Here's the drawing with two shaded views (mm, measured from the low corner). I have some questions. Give positions to 0.01 mm unless a question says otherwise; leave off trailing zeros. Write each loop counter-clockwise with the first axis right and the second up, starting at its lowest first coordinate (ties: lowest second). Pieces come first, ordered by that corner, then holes. Notation, with made-up numbers: (1, 21.5) - (28, 21.5) arc R24 cw to (28, 43.5) - close; hole circle Ø2 at (22, 58.5). An arc over 180 degrees is marked (long way). Write item = value, one per line.
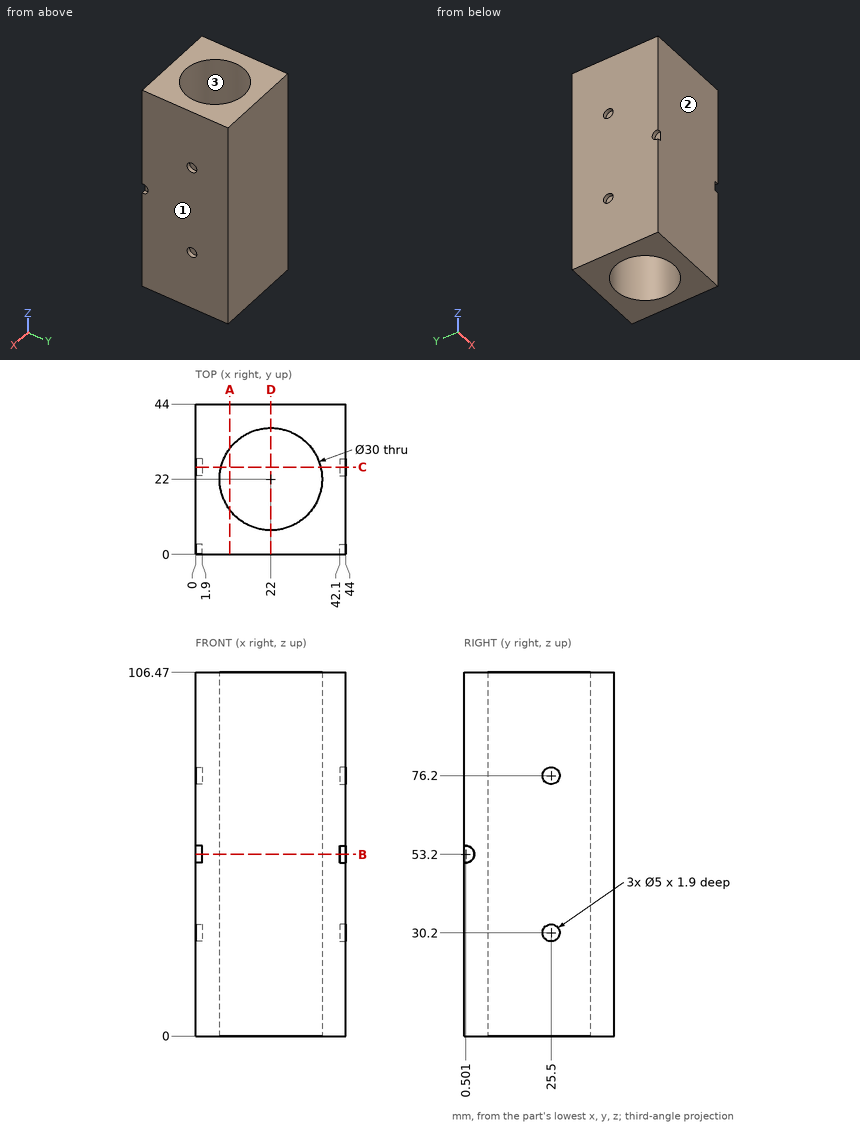
1. If we section it at B-B, the plane z = 53.2: Please give me the cut outline in (x, y), and give its area (3 significant figures).
Filled sheet:
outline = (0, 3) - (1.9, 3) - (1.9, 0) - (42.1, 0) - (42.1, 3) - (44, 3) - (44, 44) - (0, 44) - close; hole circle Ø30 at (22, 22)
area = 1,220 mm2
2. I need wall thicknesses on line 1 (Y direction, x = 22, z = 54); line 2 (Y direction, x = 13, z = 55); line 3 (X direction, y = 19.5, z = 51.5). Which ranges of each line are inside material? Lowest first, please.
Filled sheet:
line_1 = 0 to 7, 37 to 44
line_2 = 0 to 10, 34 to 44
line_3 = 0 to 7.21, 36.79 to 44
3. If we section it at C-C, the plane y = 25.5: Please give me the cut outline in (x, z).
Filled sheet:
outline = (0, 0) - (7.41, 0) - (7.41, 106.47) - (0, 106.47) - (0, 78.7) - (1.9, 78.7) - (1.9, 73.7) - (0, 73.7) - (0, 32.7) - (1.9, 32.7) - (1.9, 27.7) - (0, 27.7) - close; (36.59, 0) - (44, 0) - (44, 27.7) - (42.1, 27.7) - (42.1, 32.7) - (44, 32.7) - (44, 73.7) - (42.1, 73.7) - (42.1, 78.7) - (44, 78.7) - (44, 106.47) - (36.59, 106.47) - close
4. For pin 1 (4 mm diameter, centred on y = 0.5, z = 53.2, fed in from -X); pin 2 (2.5 mm diameter, centred on y = 25.5, z = 75.5, fed in from +X), each with a flat end and sliding along its axis, tell me the tip position at first contact or that it passes through.
Filled sheet:
pin_1 = 1.9
pin_2 = 42.1
5. Thinking about a two-plate mould opening in Y: for the marked faces 1, 2 and 3, which applies, pulls with the +Y half, pulls with the -Y half, needs draft (parallel to the pull), parting line crosses it, or undercut?
Filled sheet:
face_1 = needs draft
face_2 = pulls with the -Y half
face_3 = undercut
6. If we section it at D-D, the plane x = 22: Please give me the cut outline in (y, z).
Filled sheet:
outline = (0, 0) - (7, 0) - (7, 106.47) - (0, 106.47) - close; (37, 0) - (44, 0) - (44, 106.47) - (37, 106.47) - close
7. If we section it at A-A, the plane x = 10: Please give me the cut outline in (y, z), and give its area (3 significant figures).
Filled sheet:
outline = (0, 0) - (13, 0) - (13, 106.47) - (0, 106.47) - close; (31, 0) - (44, 0) - (44, 106.47) - (31, 106.47) - close
area = 2,770 mm2
